For this review, take the finished solid that the model builds, in its own axes (mm). A direction names the side the tool comes from. Give positions to 0.01 mm unless a question says otherwise; leave off trailing zeros. Write each loop counter-clockwise with the first axis right and the second up, starting at its lowest first coordinate (ties: lowest second). Pieces come first, ordered by that corner, then holes. Notation, with made-up numbers: M -24.5,89.5 L 24.5,89.5 A21 ccw 24.5,124.5 Z; hole C -18.75,67 d2. An arc over 180 degrees is marked long. Answer as a JSON object with one key per item and string values. Group by question number.
```python
from build123d import *

# Parameters (mm, degrees)
EXTRUDE_2_DEPTH     = 30
SKETCH_4_R          = 15
CUT_EXTRUDE_1_DEPTH = 210
SKETCH_5_R          = 15
EXTRUDE_3_DEPTH     = 10
FILLET_1_R          = 4


with BuildPart() as part:
    # 스케치3 → 보스-돌출2 (new, symmetric)
    with BuildSketch(Plane.XY):
        Polygon((0, -30), (0, 30), (15, 100), (15, 105), (-50, 105), (-50, 100), (9.886492477, 100), (-5, 30.529701772), (-5, -30.529701772), (9.886492477, -100), (-50, -100), (-50, -105), (15, -105), (15, -100), align=None)
    extrude(amount=EXTRUDE_2_DEPTH, both=True)

    # 스케치4 → 컷-돌출1 (cut)
    with BuildSketch(Plane(origin=(0, 105, 0), x_dir=(1, 0, 0), z_dir=(0, 1, 0))):
        with Locations(Location((-20, 0, 0), (0, 0, 180))):
            Circle(SKETCH_4_R)
        with BuildLine():
            Line((-20, 30), (-20, 33.122933613))
            Line((-20, 33.122933613), (-53.393516075, 33.122933613))
            Line((-53.393516075, 33.122933613), (-53.393516075, -32.957525704))
            Line((-53.393516075, -32.957525704), (-20, -32.957525704))
            Line((-20, -32.957525704), (-20, -30))
            ThreePointArc((-20, -30), (-50, 0), (-20, 30))
        make_face()
    extrude(amount=-CUT_EXTRUDE_1_DEPTH, mode=Mode.SUBTRACT)

    # 스케치5 → 보스-돌출3 (add, symmetric)
    with BuildSketch(Plane.ZY.offset(5)):
        Circle(SKETCH_5_R)
    extrude(amount=EXTRUDE_3_DEPTH, both=True)

    # 필렛1
    fillet_1_edges = [part.edges().sort_by_distance(p)[0] for p in [
        (-15, 0, -15),
    ]]
    fillet(fillet_1_edges, radius=FILLET_1_R)


solid = part.part
```
Item 1: Insertion check: P1, Ø10, axis at y = -65.5, z = -5, coming from the -X side; P2, Ø1.5, axis at x = -2, y = 53, coming from the +Z side; P3, Ø17.5, axis at y = 2.5, z = -3.5, coming from the -X side; P4, Ø10, axis at y = -73.5, z = 20, coming from the -X side. Each pin has a flat end and moves straight along its axis. Give the tip position at first contact, or say it passes through.
Item 2: Machinability: for faces 1 (the cylindrical face through (-5.015, -102.465, 0.66)), 2 (the cylindrical face through (-5.015, 102.535, 0.66)), 3 (the flat face through (2.547, 65.751, 0.42)), which of the approach directions +Z, -Z, +X, -X, +Y, -Y give a long, thin tool a straight path to every point of the face, cutting with its end or side? Answer none if there is none.
Item 3: To check wall thickness, follow probe 1 along Z at (x, y) = (-20, 102.1); probe 2 along Y at (x, z) = (-37, 4); probe 3 along Y at (x, z) = (-7.5, -12). State the ranges of each line that lie inside material, in increasing order.
Item 4: Consider section B-B (x = -44). Give the boundary of the cut face in (y, z).
Item 5: Consider section C-C (z = -24). Give the boundary of the cut face in (x, y).
Item 6: Consider section A-A (z = 0). State how many separate pieces and enclosed holes the cut face has, plus the area to 3 significant figures.
Item 7: Draft analysis for pull direction Y (two halves, no side actions). For faces 4 (the flat face through (-3, 105, 0)), 5 (the cylindrical face through (-49.993, 102.535, 0.66)), 6 (the flat face through (2.34, -64.78, 0.42)), 7 (the flat face through (-4, -105, 0)), state which applies: released by +Y, released by -Y, zero draft, split by the parting line, or undercut.
Item 8: Consider section D-D (y = 0). Give the boundary of the cut face in (x, z).
Result set:
{
 "1": {"P1": "stops at x = 1.42", "P2": "passes through", "P3": "stops at x = -15", "P4": "stops at x = 3.14"},
 "2": {"face 1": "-Y", "face 2": "+Y", "face 3": "+Z, -Z, -X"},
 "3": {"probe 1": "z = -30 to -15, 15 to 30", "probe 2": "y = -105 to -100, 100 to 105", "probe 3": "y = -105 to -100, -9 to 9, 100 to 105"},
 "4": {"outline": "M -105,-18 L -100,-18 L -100,18 L -105,18 Z; M 100,-18 L 105,-18 L 105,18 L 100,18 Z"},
 "5": {"outline": "M -38,-105 L 15,-105 L 15,-100 L 0,-30 L 0,30 L 15,100 L 15,105 L -38,105 L -38,100 L 9.89,100 L -5,30.53 L -5,-30.53 L 9.89,-100 L -38,-100 Z"},
 "6": {"separate pieces": "3", "enclosed holes": "0", "area": "1,810 mm^2"},
 "7": {"face 4": "released by +Y", "face 5": "zero draft", "face 6": "undercut", "face 7": "released by -Y"},
 "8": {"outline": "M -15,-11 A4 ccw -11,-15 L -5,-15 L -5,-30 L 0,-30 L 0,-15 L 5,-15 L 5,15 L 0,15 L 0,30 L -5,30 L -5,15 L -11,15 A4 ccw -15,11 Z"}
}
